Autodesk Fusion 360 part; units mm, degrees
sketch "Sketch1" plane through (0, 0, 0) normal (0, 0, 1) x (1, 0, 0)
  line L0 (10.1, -17.15) -> (-10.1, -17.15)
  line L1 (-10.1, -17.15) -> (-10.1, 17.15)
  line L2 (-10.1, 17.15) -> (10.1, 17.15)
  line L3 (10.1, 17.15) -> (10.1, -17.15)
  line L4 (10.1, -17.15) -> (-10.1, 17.15) construction
  line L5 (-10.1, -17.15) -> (10.1, 17.15) construction
  line L6 (11.1, 18.15) -> (-11.1, 18.15)
  line L7 (-11.1, 18.15) -> (-11.1, -18.15)
  line L8 (-11.1, -18.15) -> (11.1, -18.15)
  line L9 (11.1, -18.15) -> (11.1, 18.15)
  line L10 (11.1, 18.15) -> (-11.1, -18.15) construction
  line L11 (-11.1, 18.15) -> (11.1, -18.15) construction
  dimension "d1" = 20.2
  dimension "d2" = 34.3
  dimension "d4" = 1
  dimension "d5" = 1
extrude "Extrude1" add sketch "Sketch1" along normal blind 7
sketch "Sketch2" plane through (0, 0, 0) normal (0, 0, -1) x (1, 0, 0)
  line L0 (10.1, -17.15) -> (-10.1, -17.15)
  line L1 (-10.1, -17.15) -> (-10.1, 17.15)
  line L2 (-10.1, 17.15) -> (10.1, 17.15)
  line L3 (10.1, 17.15) -> (10.1, -17.15)
  line L4 (11.1, -18.15) -> (11.1, 18.15)
  line L5 (11.1, 18.15) -> (-11.1, 18.15)
  line L6 (-11.1, 18.15) -> (-11.1, -18.15)
  line L7 (-11.1, -18.15) -> (11.1, -18.15)
  line L8 (-11.1, 18.15) -> (11.1, 18.15)
  line L9 (11.1, 18.15) -> (11.1, -18.15)
  line L10 (11.1, -18.15) -> (-11.1, -18.15)
  line L11 (-11.1, -18.15) -> (-11.1, 18.15)
extrude "Extrude2" add sketch "Sketch2" along normal blind 0.8 contours L0 L1 L2 L3 | L4 L5 L6 L7 L8 L9 L10 L11
sketch "Sketch3" plane through (0, -18.15, 0) normal (0, -1, 0) x (1, 0, 0)
  line L0 (11.1, -0.8) -> (11.1, 7)
  line L1 (11.1, 7) -> (-11.1, 7)
  line L2 (-11.1, 7) -> (-11.1, -0.8)
  line L3 (-11.1, -0.8) -> (11.1, -0.8)
  line L4 (-5.52, 7) -> (4.08, 7)
  line L5 (4.08, 7) -> (4.08, 5.2)
  line L6 (4.08, 5.2) -> (-5.52, 5.2)
  line L7 (-5.52, 5.2) -> (-5.52, 7)
  dimension "d10" = 6
  dimension "d11" = 5.58
  dimension "d14" = 9.6
extrude "Extrude3" cut sketch "Sketch3" against normal up to surface (1 mm away) contours L1 L4 L5 L6 L7
fillet "Fillet1" radius 1.3 2 edges at (-5.52, -17.65, 5.2) (4.08, -17.65, 5.2)
sketch "Sketch4" plane through (-11.1, 0, 0) normal (-1, 0, 0) x (0, -1, 0)
  line L0 (18.15, -0.8) -> (18.15, 7)
  line L1 (18.15, 7) -> (-18.15, 7)
  line L2 (-18.15, 7) -> (-18.15, -0.8)
  line L3 (-18.15, -0.8) -> (18.15, -0.8)
  line L4 (9.95, 6.65) -> (14.95, 6.65)
  line L5 (14.95, 6.65) -> (14.95, 5.45)
  line L6 (14.95, 5.45) -> (9.95, 5.45)
  line L7 (9.95, 5.45) -> (9.95, 6.65)
  dimension "d17" = 3.2
  dimension "d18" = 5
  dimension "d19" = 1.2
  dimension "d22" = 0.35
extrude "Extrude4" cut sketch "Sketch4" against normal up to surface (1 mm away) contours L4 L5 L6 L7
fillet "Fillet2" radius 0.15 4 edges at (-11.1, -12.45, 5.45) (-11.1, -9.95, 6.05) (-11.1, -12.45, 6.65) (-11.1, -14.95, 6.05)
sketch "Sketch5" plane through (0, 0, 7) normal (0, 0, 1) x (-1, 0, 0)
  line L0 (-4.08, 17.15) -> (-4.08, 18.15)
  line L1 (-4.08, 18.15) -> (-11.1, 18.15)
  line L2 (-11.1, 18.15) -> (-11.1, -18.15)
  line L3 (-11.1, -18.15) -> (11.1, -18.15)
  line L4 (11.1, -18.15) -> (11.1, 18.15)
  line L5 (11.1, 18.15) -> (5.52, 18.15)
  line L6 (5.52, 18.15) -> (5.52, 17.15)
  line L7 (5.52, 17.15) -> (10.1, 17.15)
  line L8 (10.1, 17.15) -> (10.1, -17.15)
  line L9 (10.1, -17.15) -> (-10.1, -17.15)
  line L10 (-10.1, -17.15) -> (-10.1, 17.15)
  line L11 (-10.1, 17.15) -> (-4.08, 17.15)
  line L12 (10.6, -17.65) -> (-10.6, -17.65)
  line L13 (-10.6, -17.65) -> (-10.6, 17.65)
  line L14 (-10.6, 17.65) -> (10.6, 17.65)
  line L15 (10.6, 17.65) -> (10.6, -17.65)
  dimension "d26" = 0.5
  dimension "d27" = 0.5
  dimension "d28" = 0.5
  dimension "d29" = 0.5
extrude "Extrude5" add sketch "Sketch5" along normal blind 1.5 contours L0 L6 L7 L8 L9 L10 L11 L12 L13 L14 L15
sketch "Sketch7" plane through (10.6, 0, 0) normal (1, 0, 0) x (0, 1, 0)
  line L0 (-17.65, 7) -> (17.65, 7)
  line L1 (17.65, 7) -> (17.65, 8.5)
  line L2 (17.65, 8.5) -> (-17.65, 8.5)
  line L3 (-17.65, 8.5) -> (-17.65, 7)
  line L4 (-17.65, 8.5) -> (17.65, 7) construction
  line L5 (17.65, 8.5) -> (-17.65, 7) construction
  line L6 (0, 7.75) -> (-14.5, 7.75) construction
  line L7 (7.5, 7.45) -> (-7.5, 7.45)
  line L8 (-7.5, 7.45) -> (-7.5, 8.05)
  line L9 (-7.5, 8.05) -> (7.5, 8.05)
  line L10 (7.5, 8.05) -> (7.5, 7.45)
  line L11 (7.5, 7.45) -> (-7.5, 8.05) construction
  line L12 (-7.5, 7.45) -> (7.5, 8.05) construction
  point P0 (0, 7.75)
  dimension "d32" = 15
  dimension "d33" = 0.6
ref_plane "WorkPlane1" through (0, 0, 7.75) normal (1, 0, 0) x (0, 1, 0)
extrude "Extrude6" cut sketch "Sketch7" against normal blind 0.2 contours L7 L8 L9 L10
fillet "Fillet5" radius 0.2 4 edges at (10.5, -7.5, 7.45) (10.5, -7.5, 8.05) (10.5, 7.5, 7.45) (10.5, 7.5, 8.05)
fillet "Fillet6" radius 0.2 8 edges at (10.6, -7.4414, 7.5086) (10.6, 0, 7.45) (10.6, 7.4414, 7.5086) (10.6, 7.5, 7.75) (10.6, 7.4414, 7.9914) (10.6, 0, 8.05) (10.6, -7.4414, 7.9914) (10.6, -7.5, 7.75)
mirror "Mirror2" about plane through (0, 0, 7.75) normal (1, 0, 0) of "Extrude6"
fillet "Fillet7" radius 0.2 4 edges at (-10.5, 7.5, 7.45) (-10.5, 7.5, 8.05) (-10.5, -7.5, 7.45) (-10.5, -7.5, 8.05)
fillet "Fillet8" radius 0.2 8 edges at (-10.6, -7.4414, 7.9914) (-10.6, -7.5, 7.75) (-10.6, -7.4414, 7.5086) (-10.6, 0, 7.45) (-10.6, 7.4414, 7.5086) (-10.6, 7.5, 7.75) (-10.6, 7.4414, 7.9914) (-10.6, 0, 8.05)
fillet "Fillet9" radius 0.5 8 edges at (-11.1, 18.15, 3.1) (-11.1, -18.15, 3.1) (-11.1, 0, -0.8) (0, -18.15, -0.8) (11.1, -18.15, 3.1) (11.1, 0, -0.8) (11.1, 18.15, 3.1) (0, 18.15, -0.8)
sketch "Sketch8" plane through (0, 17.15, 0) normal (0, -1, 0) x (1, 0, 0)
  line L0 (-10.1, 0) -> (10.1, 0)
  line L1 (10.1, 0) -> (10.1, 8.5)
  line L2 (10.1, 8.5) -> (-10.1, 8.5)
  line L3 (-10.1, 8.5) -> (-10.1, 0)
  line L4 (4, 6.5) -> (5.5, 6.5)
  line L5 (5.5, 6.5) -> (5.5, 5.5)
  line L6 (5.5, 5.5) -> (4, 5.5)
  line L7 (4, 5.5) -> (4, 6.5)
  dimension "d55" = 4.6
  dimension "d56" = 2
  dimension "d57" = 1.5
  dimension "d58" = 1
extrude "Extrude7" cut sketch "Sketch8" against normal up to surface (1 mm away) contours L4 L5 L6 L7
fillet "Fillet10" radius 0.3 4 edges at (5.5, 17.65, 5.5) (5.5, 17.65, 6.5) (4, 17.65, 6.5) (4, 17.65, 5.5)
equation "case_thickness = 1 mm"
equation "d4 = case_thickness"
equation "d5 = case_thickness"
equation "d8 = case_bottom - 0.2 mm"
equation "d11 = 4.58 mm + case_thickness"
equation "lock_rim = 0.5 mm"
equation "d26 = lock_rim"
equation "d27 = lock_rim"
equation "d28 = lock_rim"
equation "d29 = lock_rim"
equation "d43 = clip_roundness"
equation "d45 = clip_roundness"
equation "clip_roundness = 0.2 mm"
equation "d50 = clip_roundness"
equation "d52 = clip_roundness"
equation "case_bottom = 1 mm"
Design review of the part built by this model. Coordinates are the model's own, in mm. A direction names the side the tool comes from. Coordinates: 2 decimals unless noted, no trailing zeros. Order: outer loops, then holes, each group sorted by start corner. A loop starts at its lowest first (then second) coordinate and runs counter-clockwise, first axis right, second up. Notation, with made-up numbers: (10.5, 75.25) - (48.5, 75.25) arc R24 ccw to (48.5, 109.25) - close; hole circle Ø3 at (-35, 28). An arc over 180 degrees is marked (long way). One line per question, with ' | ' between items.
Q1. Consider section C-C, the plane x = 0.75. Give the boundary of the cut face in (y, z).
Answer key:
outline: (-18.15, -0.3) arc R0.5 ccw to (-17.65, -0.8) - (17.65, -0.8) arc R0.5 ccw to (18.15, -0.3) - (18.15, 7) - (17.65, 7) - (17.65, 8.5) - (17.15, 8.5) - (17.15, 0) - (-17.15, 0) - (-17.15, 5.2) - (-18.15, 5.2) - close
Q2. The part is to be moulded in two halves that separate along X. For faces 1 (the flat face through (0, -17.15, 3)), 2 (the flat face through (-11.1, 0, 3)), 3 (the flat face through (0, 18.15, 3)), say which applies: +X half, -X half, draft (parallel to the pull), parting line (faces both ways), or undercut.
Answer key:
face 1: undercut | face 2: -X half | face 3: draft
Q3. For faces 4 (the flat face through (-10.5, -12.4, 6.65)), 5 (the flat face through (4.08, -17.4, 7.3)), 6 (the flat face through (4.8, 17.6, 5.5)), 7 (the flat face through (-8, -17.65, 8)), 8 (the flat face through (-10.1, 0, 4)), list the 3-axis set-ups (+Z, -Z, +X, -X, +Y, -Y) from which the entire face can be reached by the end or side of a thin tool; tool diameter is ignored.
Answer key:
face 4: -X | face 5: +Z, -Y | face 6: +Y | face 7: +Z, +X, -X, -Y | face 8: +Z
Q4. To check wall thickness, follow line 1 along Y through (x, z) = (-6, 4.25); line 2 along X through (y, z) = (2.5, 2.75); line 3 along Y through (x, z) = (-6.25, 8.25). State the ranges of each line that lie inside material, in increasing order.
Answer key:
line 1: y = -18.15 to -17.15, 17.15 to 18.15 | line 2: x = -11.1 to -10.1, 10.1 to 11.1 | line 3: y = -17.65 to -17.15, 17.15 to 17.65
Q5. Consider section B-B, the plane z = 4.5. Give the boundary of the cut face in (x, y), then the cut area to 3 significant figures.
Answer key:
outline: (-11.1, -17.65) arc R0.5 ccw to (-10.6, -18.15) - (10.6, -18.15) arc R0.5 ccw to (11.1, -17.65) - (11.1, 17.65) arc R0.5 ccw to (10.6, 18.15) - (-10.6, 18.15) arc R0.5 ccw to (-11.1, 17.65) - close; hole (-10.1, -17.15) - (10.1, -17.15) - (10.1, 17.15) - (-10.1, 17.15) - close | area: 113 mm2
Q6. Clearance check with flat-ended pins moving along their axes: pin 1 Ø1.6 at (x, z) = (8.5, 8) entering from -Y; pin 2 Ø12 at (x, y) = (2, -7.5) entering from +Z; pin 3 Ø1.6 at (y, z) = (-3.5, 8) entering from +X. State where each tip first meets the part, or that it passes through.
Answer key:
pin 1: stops at y = -17.65 | pin 2: stops at z = 0 | pin 3: stops at x = 10.6
Q7. Consider section A-A, the plane y = -12.5. Give the boundary of the cut face in (x, z), then the cut area to 3 significant figures.
Answer key:
outline: (-11.1, -0.3) arc R0.5 ccw to (-10.6, -0.8) - (10.6, -0.8) arc R0.5 ccw to (11.1, -0.3) - (11.1, 7) - (10.6, 7) - (10.6, 8.5) - (10.1, 8.5) - (10.1, 0) - (-10.1, 0) - (-10.1, 5.45) - (-10.95, 5.45) arc R0.15 ccw to (-11.1, 5.3) - close; (-11.1, 6.8) arc R0.15 ccw to (-10.95, 6.65) - (-10.1, 6.65) - (-10.1, 8.5) - (-10.6, 8.5) - (-10.6, 7) - (-11.1, 7) - close | area: 31.9 mm2
Q8. Consider section D-D, the plane y = 13. Give the boundary of the cut face in (x, z).
Answer key:
outline: (-11.1, -0.3) arc R0.5 ccw to (-10.6, -0.8) - (10.6, -0.8) arc R0.5 ccw to (11.1, -0.3) - (11.1, 7) - (10.6, 7) - (10.6, 8.5) - (10.1, 8.5) - (10.1, 0) - (-10.1, 0) - (-10.1, 8.5) - (-10.6, 8.5) - (-10.6, 7) - (-11.1, 7) - close
